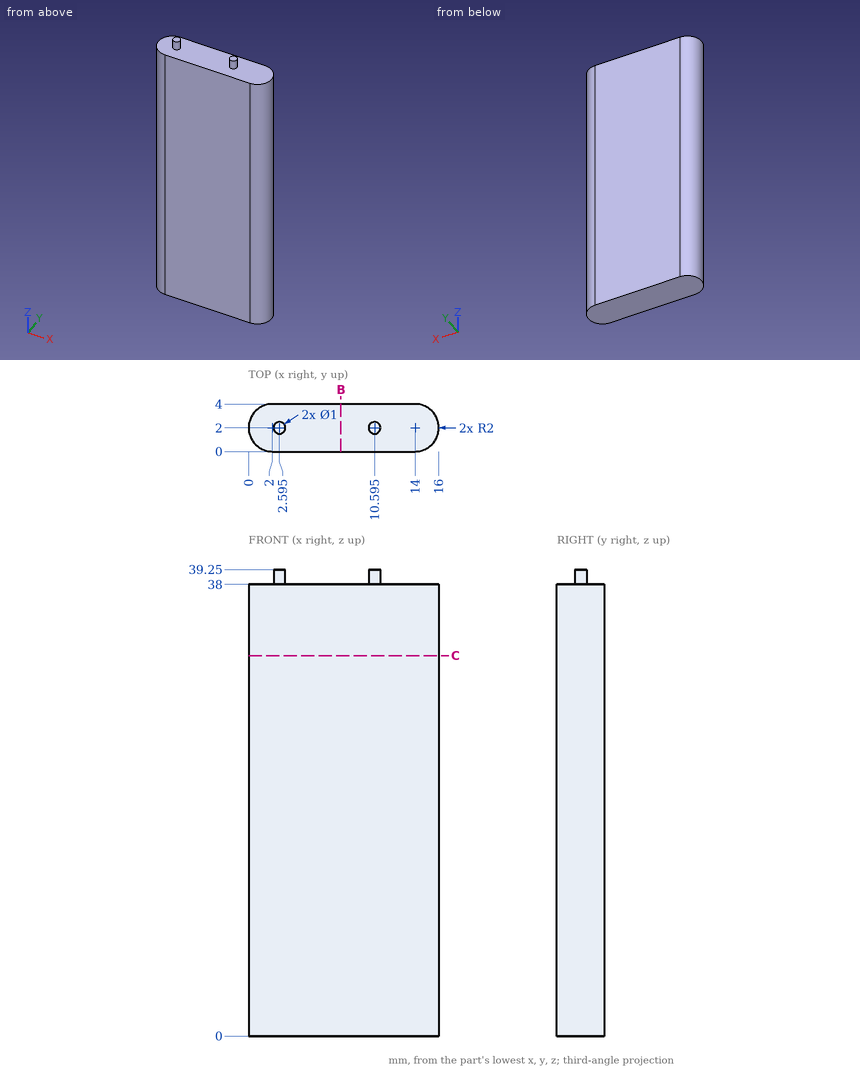
Print and shaded views of the part. All mm, measured from the part's lowest x, y and z. Coordinates: 2 decimals unless noted, no trailing zeros. Order: outer loops, then holes, each group sorted by start corner. A loop starts at its lowest first (then second) coordinate and runs counter-clockwise, first axis right, second up. Notation, with made-up numbers: M 73.5,16.5 L 130.5,16.5 A20 cw 130.5,33.5 Z; hole C -1,32 d4. An arc over 180 degrees is marked long. One line per question, with ' | ' between items. Start each with the question number.
Q1. Flat gauge pins, fed straight in: pin 1 Ø2 at (y, z) = (1.5, 29.5) entering from -X; pin 2 Ø2 at (y, z) = (3.5, 16) entering from +X; pin 3 Ø1.2 at (x, y) = (8, 2.5) entering from +Z. Where does each tip first touch, or does it go through?
Q2. Saw through at B-B (x = 7.75). List the corners of the cut face in (y, z), then the cut area to 3 significant figures.
Q3. Saw through at C-C (z = 32). List the corners of the cut face in (x, y).
Q4. Probe L1, parallel to Z at x = 7.5, y = 0.6; L2, parallel to X at y = 1.9, z = 32; L3, parallel to X at y = 3.45, z = 16. List the from-to ranges inside material, lowest first. Write a range as from..to.
Check values:
1) pin 1: stops at x = 0 | pin 2: stops at x = 15.94 | pin 3: stops at z = 38
2) outline: M 0,0 L 4,0 L 4,38 L 0,38 Z | area: 152 mm2
3) outline: M 2,0 L 14,0 A2 ccw 14,4 L 2,4 A2 ccw Z
4) L1: z = 0..38 | L2: x = 0..16 | L3: x = 0.62..15.38
